from build123d import *

# Parameters (mm, degrees)
F0_R     = 3.81
F1_DEPTH = 3.81
F2_R     = 5.715
F3_DEPTH = 1.5748


with BuildPart() as f1:
    # F0 (on Front) → F1 (new body)
    with BuildSketch(Plane.XZ):
        Circle(F0_R)
    extrude(amount=F1_DEPTH)

    # F2 (on face) → F3 (join)
    with BuildSketch(Plane(origin=(0, 0, 0), x_dir=(-1, 0, 0), z_dir=(0, 1, 0))):
        Circle(F2_R)
    extrude(amount=F3_DEPTH)

    # F4 (on Right) → F5 (revolve, cut)
    with BuildSketch(Plane.YZ):
        Polygon((-3.879813, 1.5875), (-3.879813, 0), (1.65217, 0), (1.65217, 2.562938), align=None)
    revolve(axis=Axis((0, -1.113821, 0), (0, 1, 0)), mode=Mode.SUBTRACT)


solid = f1.part
Geometry check sheet. Reference: the model listing, model coordinates, mm. A direction names the side the tool comes from. Round coordinates to 2 decimals unless told otherwise and drop trailing zeros. Loops run counter-clockwise (first coordinate to the right, second up) from the corner with the lowest first, then second, coordinate; pieces in that order, holes last. Notation, with made-up numbers: (84, 0.5) -> (88, 0.5) arc R19 ccw to (88, 8.5) -> close; hole circle Ø9 at (15, -13.75). An arc over 180 degrees is marked (long way). Answer as a JSON object with one key per item and string values. Group by question number.
Item 1: Set-up check for faces 4 (the face through (-5.45, 0.78, 1.72)), 5 (the face through (-1, 0, -4)): record each of +Z, -Z, +X, -X, +Y, -Y from which the full face is reachable in a straight line by a thin tool's end or side.
Item 2: Cross-section at B-B, the plane x = 0. Record the cut outline in (y, z) (3 decimals).
Item 3: Cross-section at A-A, the plane z = 0. Record the cut outline in (x, y) (3 decimals), plus the area to 3 significant figures.
Item 4: Release check for a two-part mould opening along X. For faces 1 (the face through (-1.2, 1.575, -2.5)), 2 (the face through (0.589, -1.754, 1.872)), 3 (the face through (-0.83, -1.88, -3.72)) record: pulls with the +X half, pulls with the -X half, needs draft (parallel to the pull), parting line crosses it, or undercut.
Item 5: Depth check by flat-ended pin: pin 1 Ø3 at (x, y) = (0, -2) entering from +Z; pin 2 Ø1.5 at (x, y) = (-3, -3) entering from +Z; pin 3 Ø1.5 at (y, z) = (0, 2) entering from +X. Enter the tip coordinate at first touch or a pass-through.
Item 6: Thickness scan on line 1 along Y through (x, z) = (5, 0.5); line 2 along Z through (x, y) = (1.75, -1.55); line 3 along X through (y, z) = (-0.95, -0.5). Record the ranges inside material, lowest first.
Item 7: Cross-section at D-D, the plane y = -1.3. Record the cut outline in (x, z).
Item 8: Cross-section at C-C, the plane x = -3.25. Record the cut outline in (y, z), plus the area to 3 significant figures.
Determined:
{
 "1": {"face 4": "+Y, -Y", "face 5": "-Y"},
 "2": {"outline": "(-3.81, -3.81) -> (0, -3.81) -> (0, -5.715) -> (1.575, -5.715) -> (1.575, -2.549) -> (-3.81, -1.6) -> close; (-3.81, 1.6) -> (1.575, 2.549) -> (1.575, 5.715) -> (0, 5.715) -> (0, 3.81) -> (-3.81, 3.81) -> close"},
 "3": {"outline": "(-5.715, 0) -> (-3.81, 0) -> (-3.81, -3.81) -> (-1.6, -3.81) -> (-2.549, 1.575) -> (-5.715, 1.575) -> close; (1.6, -3.81) -> (3.81, -3.81) -> (3.81, 0) -> (5.715, 0) -> (5.715, 1.575) -> (2.549, 1.575) -> close", "area": "24.7 mm²"},
 "4": {"face 1": "needs draft", "face 2": "undercut", "face 3": "parting line crosses it"},
 "5": {"pin 1": "stops at z = 3.81", "pin 2": "stops at z = 3.07", "pin 3": "stops at x = 5.58"},
 "6": {"line 1": "y = 0 to 1.57", "line 2": "z = -3.38 to -0.96, 0.96 to 3.38", "line 3": "x = -3.78 to -2.04, 2.04 to 3.78"},
 "7": {"outline": "circle Ø7.62 at (0, 0); hole circle Ø4.08 at (0, 0)"},
 "8": {"outline": "(-3.81, -1.99) -> (0, -1.99) -> (0, -4.7) -> (1.57, -4.7) -> (1.57, 4.7) -> (0, 4.7) -> (0, 1.99) -> (-3.81, 1.99) -> close", "area": "30.0 mm²"}
}
